Work out the finished part from the listing and answer in its coordinate system (mm). A direction names the side the tool comes from. Coordinates: 2 decimals unless noted, no trailing zeros. Write each loop counter-clockwise with the first axis right and the second up, starting at its lowest first coordinate (ties: lowest second). Pieces come first, ordered by that corner, then holes. Notation, with made-up numbers: (75, -12.75) -> (101, -12.75) arc R29 cw to (101, 25.25) -> close; hole circle Ø3 at (-34.5, 36). An arc over 180 degrees is marked (long way). Write each question's results on one line, items separated by ' | '. Start each with the question number.
from build123d import *

# Parameters (mm, degrees)
SKETCH_1_W      = 50
SKETCH_1_H      = 20
SKETCH_1_W_2    = 30
SKETCH_1_H_2    = 15
EXTRUDE_1_DEPTH = 285
SKETCH_2_R      = 10
EXTRUDE_2_DEPTH = 30
SKETCH_3_R      = 5
EXTRUDE_3_DEPTH = 30


with BuildPart() as part:
    # Эскиз1 → Бобышка-Вытянуть1 (new, symmetric)
    with BuildSketch(Plane.XY):
        Rectangle(SKETCH_1_W, SKETCH_1_H)
        Rectangle(SKETCH_1_W_2, SKETCH_1_H_2, mode=Mode.SUBTRACT)
    extrude(amount=EXTRUDE_1_DEPTH, both=True)

    # Эскиз2 → Бобышка-Вытянуть2 (add)
    with BuildSketch(Plane.XZ.offset(10)):
        with Locations(Location((0, 260, 0), (0, 0, 90))):
            Circle(SKETCH_2_R)
        with Locations(Location((0, -260, 0), (0, 0, 90))):
            Circle(SKETCH_2_R)
    extrude(amount=EXTRUDE_2_DEPTH)

    # Эскиз3 → Бобышка-Вытянуть3 (add)
    with BuildSketch(Plane(origin=(0, 10, 0), x_dir=(1, 0, 0), z_dir=(0, 1, 0))):
        with Locations(Location((0, 59, 0), (0, 0, 90))):
            Circle(SKETCH_3_R)
    extrude(amount=EXTRUDE_3_DEPTH)


solid = part.part
1. Find section C-C on z = 260. Give the vertices of the cut face in (x, y).
2. For faces 4 (the face through (0, 9, 285)), 5 (the face through (3.83, -24.79, -250.763)), 6 (the face through (-15, 0, 4)), determine the directions among +Z, -Z, +X, -X, +Y, -Y from which every point of the face is accessible in a straight line to the end or side of a thin tool.
3. Given pin 1 Ø1 at (x, z) = (-13.5, -99) entering from -Y; pin 2 Ø15 at (x, z) = (0.5, 138.5) entering from +Y; pin 3 Ø12 at (x, y) = (-5.5, 31) entering from +Z, each flat-ended and moving along its own axis, determine where each tip first touches the part or whether it passes through.
4. Find the intervals of material crossed by L1, parallel to Y at x = 10.5, z = -32; L2, parallel to X at y = -6.5, z = -52.5; L3, parallel to Z at x = -2, y = -31, in increasing order.
5. Find section B-B on x = 0. Give the vertices of the cut face in (y, z), and give its area (3 significant figures).
6. Determine the mould class of faces 1 (the face through (25, 0, 4)), 2 (the face through (-3, -24.79, 269.54)), 3 (the face through (0, 25, -54)) for opening direction Z: pulls with the +Z half, pulls with the -Z half, needs draft (parallel to the pull), parting line crosses it, or undercut.
7. Find section D-D on y = 29. Give the vertices of the cut face in (x, z).
8. Find section A-A on z = -59. Give the vertices of the cut face in (x, y).
Ans:
1) outline: (-25, -10) -> (-10, -10) -> (-10, -40) -> (10, -40) -> (10, -10) -> (25, -10) -> (25, 10) -> (-25, 10) -> close; hole (-15, -7.5) -> (15, -7.5) -> (15, 7.5) -> (-15, 7.5) -> close
2) face 4: +Z, +X, -X, +Y, -Y | face 5: -Y | face 6: +Z, -Z
3) pin 1: stops at y = -10 | pin 2: stops at y = 10 | pin 3: stops at z = -54
4) L1: y = -10 to -7.5, 7.5 to 10 | L2: x = -25 to -15, 15 to 25 | L3: z = -269.8 to -250.2, 250.2 to 269.8
5) outline: (-40, -270) -> (-10, -270) -> (-10, -285) -> (-7.5, -285) -> (-7.5, 285) -> (-10, 285) -> (-10, 270) -> (-40, 270) -> (-40, 250) -> (-10, 250) -> (-10, -250) -> (-40, -250) -> close; (7.5, -285) -> (10, -285) -> (10, -64) -> (40, -64) -> (40, -54) -> (10, -54) -> (10, 285) -> (7.5, 285) -> close | area: 4,350 mm²
6) face 1: needs draft | face 2: undercut | face 3: parting line crosses it
7) outline: circle Ø10 at (0, -59)
8) outline: (-25, -10) -> (25, -10) -> (25, 10) -> (5, 10) -> (5, 40) -> (-5, 40) -> (-5, 10) -> (-25, 10) -> close; hole (-15, -7.5) -> (15, -7.5) -> (15, 7.5) -> (-15, 7.5) -> close
